```python
from build123d import *

# Parameters (mm, degrees)
SKETCH_W      = 180
SKETCH_H      = 145
PAD_DEPTH     = 45
SKETCH001_R   = 8.128419
SKETCH001_R_2 = 8.170495
PAD001_DEPTH  = 5.3


with BuildPart() as part:
    # Sketch → Pad (new body)
    with BuildSketch(Plane.XY):
        with Locations((90, 72.5)):
            Rectangle(SKETCH_W, SKETCH_H)
    extrude(amount=PAD_DEPTH)

    # Sketch001 (on Face6 of Pad) → Pad001 (join)
    with BuildSketch(Plane.XY.offset(45)):
        with Locations((13.5, 112.5)):
            Circle(SKETCH001_R)
        with Locations((13.5, 32.5)):
            Circle(SKETCH001_R_2)
    extrude(amount=PAD001_DEPTH)


solid = part.part
```
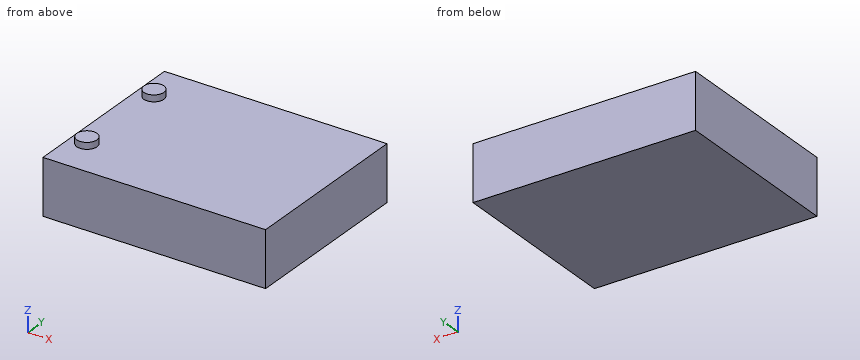
CAD build for the part. Positions are in the model's coordinates, mm. Round coordinates to 2 decimals unless told otherwise and drop trailing zeros. Loops run counter-clockwise (first coordinate to the right, second up) from the corner with the lowest first, then second, coordinate; pieces in that order, holes last. Notation, with made-up numbers: M 16.25,87.5 L 39.25,87.5 A18 cw 39.25,91.5 Z; hole C 38.5,40.25 d2. An arc over 180 degrees is marked long. Use a Markdown table: item, result. Add a question column.
(1) Drill centre lines: line 1 (Z direction, x = 85, y = 46.5); line 2 (X direction, y = 119, z = 46.5). Where is each one in solid material? Low to high.
(2) Cut at C-C (x = 63). Give the cut face in (y, z).
(3) Cut at A-A (y = 32.5). Give the cut face in (x, z), and give its area (3 significant figures).
(4) Cut at D-D (y = 112.5). Give the cut face in (x, z).
(5) Flat gauge pin, fed straight in: pin 1 (8 mm diameter, centred on x = 69.5, y = 35, fed in from +Z). Where does the tip first touch, or does it go through?
(6) Cut at B-B (z = 47.5). Give the cut face in (x, y).
Geometry says:
| question | item | result |
|---|---|---|
| 1 | line 1 | z = 0 to 45 |
| 1 | line 2 | x = 8.62 to 18.38 |
| 2 | outline | M 0,0 L 145,0 L 145,45 L 0,45 Z |
| 3 | outline | M 0,0 L 180,0 L 180,45 L 21.67,45 L 21.67,50.3 L 5.33,50.3 L 5.33,45 L 0,45 Z |
| 3 | area | 8,190 mm² |
| 4 | outline | M 0,0 L 180,0 L 180,45 L 21.63,45 L 21.63,50.3 L 5.37,50.3 L 5.37,45 L 0,45 Z |
| 5 | pin 1 | stops at z = 45 |
| 6 | outline | C 13.5,32.5 d16.34; C 13.5,112.5 d16.26 |
